Source: CAD feature listing. Evaluate the final solid. Frame: model axes, mm. Coordinates: 2 decimals unless noted, no trailing zeros. Order: outer loops, then holes, each group sorted by start corner. A loop starts at its lowest first (then second) coordinate and runs counter-clockwise, first axis right, second up.
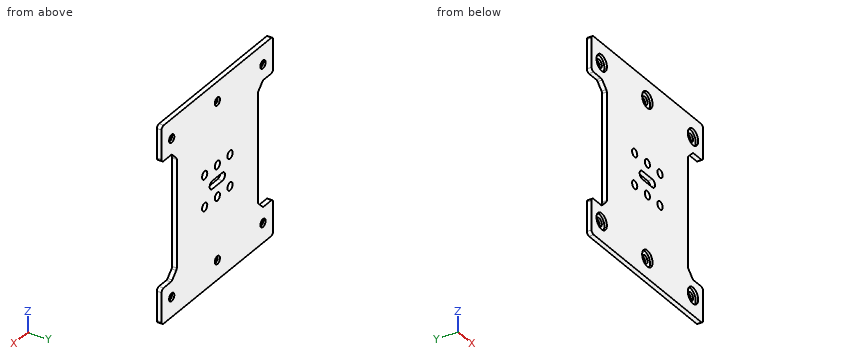
```python
from build123d import *

# Parameters (mm, degrees)
F1_DEPTH       = 3
F2_D           = 5.1
F2_DEPTH       = 34.5
F2_TIP         = 1.5321945785
F3_D           = 5.1
F3_DEPTH       = 34.5
F3_CBORE_D     = 10.2
F3_CBORE_DEPTH = 1.6
F3_TIP         = 1.5321945785
F5_D           = 5.1
F5_DEPTH       = 34.5
F5_TIP         = 1.5321945785
F6_D           = 5.1
F6_DEPTH       = 34.5
F6_CBORE_D     = 10.2
F6_CBORE_DEPTH = 1.6
F6_TIP         = 1.5321945785


# Not quite as in the source:
# - a feature names something its author has since deleted; it is built from what else it names


with BuildPart() as f1:
    # F0 (on Front) → F1 (new body)
    with BuildSketch(Plane.XZ):
        with BuildLine():
            Line((-157.7735108339, 88.9936834574), (-210.7735108339, 88.9936834574))
            ThreePointArc((-210.7735108339, 88.9936834574), (-212.1877243962, 88.4078970197), (-212.7735108339, 86.9936834574))
            Line((-212.7735108339, 86.9936834574), (-212.7735108339, 68.4936834574))
            ThreePointArc((-212.7735108339, 68.4936834574), (-212.1877243962, 67.079469895), (-210.7735108339, 66.4936834574))
            Line((-210.7735108339, 66.4936834574), (-203.5195108339, 66.4936834574))
            ThreePointArc((-203.5195108339, 66.4936834574), (-202.8306806556, 66.3566666159), (-202.2467186277, 65.9664756635))
            Line((-202.2467186277, 65.9664756635), (-198.3007186277, 62.0204756635))
            ThreePointArc((-198.3007186277, 62.0204756635), (-197.9105276754, 61.4365136356), (-197.7735108339, 60.7476834574))
            Line((-197.7735108339, 60.7476834574), (-197.7735108339, 26.4936834574))
            Line((-197.7735108339, 26.4936834574), (-165.3235108339, 26.4936834574))
            ThreePointArc((-165.3235108339, 26.4936834574), (-164.5766331259, 28.2968057494), (-162.7735108339, 29.0436834574))
            Line((-162.7735108339, 29.0436834574), (-157.7735108339, 29.0436834574))
            Line((-157.7735108339, 29.0436834574), (-157.7735108339, 88.9936834574))
        make_face()
    extrude(amount=-F1_DEPTH)

    # F2
    with Locations(Plane.XZ):
        with Locations((-170.2735108339, 36.4936834574)):
            Hole(F2_D / 2, depth=F2_DEPTH)
            with Locations((0, 0, -(F2_DEPTH + F2_TIP / 2))):  # 118° drill point
                Cone(0, F2_D / 2, F2_TIP, mode=Mode.SUBTRACT)

    # F3
    with Locations(Plane.XZ):
        with Locations((-202.7735108339, 76.4936834574)):
            CounterBoreHole(F3_D / 2, F3_CBORE_D / 2, F3_CBORE_DEPTH, depth=F3_DEPTH)
            with Locations((0, 0, -(F3_DEPTH + F3_TIP / 2))):  # 118° drill point
                Cone(0, F3_D / 2, F3_TIP, mode=Mode.SUBTRACT)

    # F4: F1 across face


with BuildPart() as f1_1:
    add(f1.part)
    add(f1.part.mirror(Plane(origin=(-157.7735108339, 1.5, 59.0186834574), x_dir=(0, 1, 0), z_dir=(1, 0, 0))))

    # F5
    with Locations(Plane.XZ):
        with Locations((-157.7735108339, 36.4936834574)):
            Hole(F5_D / 2, depth=F5_DEPTH)
            with Locations((0, 0, -(F5_DEPTH + F5_TIP / 2))):  # 118° drill point
                Cone(0, F5_D / 2, F5_TIP, mode=Mode.SUBTRACT)

    # F6
    with Locations(Plane.XZ):
        with Locations((-157.7735108339, 76.4936834574)):
            CounterBoreHole(F6_D / 2, F6_CBORE_D / 2, F6_CBORE_DEPTH, depth=F6_DEPTH)
            with Locations((0, 0, -(F6_DEPTH + F6_TIP / 2))):  # 118° drill point
                Cone(0, F6_D / 2, F6_TIP, mode=Mode.SUBTRACT)

    # F7: F1 across face


with BuildPart() as f1_2:
    add(f1_1.part)
    add(f1_1.part.mirror(Plane(origin=(-181.5485108339, 1.5, 26.4936834574), x_dir=(1, 0, 0), z_dir=(0, 0, -1))))


solid = f1_2.part
```
1. Ray query, line 1 (X direction, y = 0.8, z = -24); line 2 (X direction, y = 1.3, z = 73.5); line 3 (Z direction, x = -111, y = 0.95). Return the intervals inside material, ascending.
Findings:
line 1: x = -212.77 to -207.85, -197.7 to -162.85, -152.7 to -117.85, -107.7 to -102.77
line 2: x = -212.77 to -206.9, -198.64 to -161.9, -153.64 to -116.9, -108.64 to -102.77
line 3: z = -36.01 to -28.29, -18.72 to -13.51, 66.49 to 71.71, 81.28 to 88.99
2. Pin query (flat end, axial travel): P1, Ø5, axis at x = -156.5, z = -23.5, coming from the -Y side. Return the tip coordinate at first contact, or that it passes through.
Findings:
P1: stops at y = 1.6
3. Section query B-B on y = 0.85. Count the separate pieces of the cut face and the enclosed holes in it, plus the area to 3 significant figures.
Findings:
separate pieces: 1
enclosed holes: 13
area: 10,700 mm2
4. Section query A-A on z = 10.5. Return loops of the section in (x, y).
Findings:
outline: (-197.77, 0) - (-117.77, 0) - (-117.77, 3) - (-197.77, 3) - close
